CAD build for the part. Positions are in the model's coordinates, mm. A direction names the side the tool comes from. Give positions to 0.01 mm unless a question says otherwise; leave off trailing zeros. Loops run counter-clockwise (first coordinate to the right, second up) from the corner with the lowest first, then second, coordinate; pieces in that order, holes last.
```python
from build123d import *

# Parameters (mm, degrees)
ESQUISSE1_R        = 6.5
ESQUISSE1_R_2      = 6
ESQUISSE1_R_3      = 2.5
BOSS_EXTRU_1_DEPTH = 3
CONG_1_R           = 6


with BuildPart() as part:
    # Esquisse1 → Boss.-Extru.1 (new body)
    with BuildSketch(Plane.XY):
        with BuildLine():
            Line((0, 10), (20, 10))
            ThreePointArc((20, 10), (25.257311121, 8.506508084), (28.94427191, 4.472135955))
            Line((28.94427191, 4.472135955), (38.94427191, -15.527864045))
            ThreePointArc((38.94427191, -15.527864045), (34.472135955, -28.94427191), (21.05572809, -24.472135955))
            Line((21.05572809, -24.472135955), (13.819660113, -10))
            Line((13.819660113, -10), (6.180339887, -10))
            Line((6.180339887, -10), (-1.05572809, -24.472135955))
            ThreePointArc((-1.05572809, -24.472135955), (-14.472135955, -28.94427191), (-18.94427191, -15.527864045))
            Line((-18.94427191, -15.527864045), (-8.94427191, 4.472135955))
            ThreePointArc((-8.94427191, 4.472135955), (-5.257311121, 8.506508084), (0, 10))
        make_face()
        Circle(ESQUISSE1_R, mode=Mode.SUBTRACT)
        with Locations((20, 0)):
            Circle(ESQUISSE1_R_2, mode=Mode.SUBTRACT)
        with Locations((-10, -20)):
            Circle(ESQUISSE1_R_3, mode=Mode.SUBTRACT)
        with Locations((30, -20)):
            Circle(ESQUISSE1_R_3, mode=Mode.SUBTRACT)
    extrude(amount=BOSS_EXTRU_1_DEPTH)

    # Congé1
    cong_1_edges = [part.edges().sort_by_distance(p)[0] for p in [
        (6.180339887, -10, 1.5),
        (13.819660113, -10, 1.5),
    ]]
    fillet(cong_1_edges, radius=CONG_1_R)


solid = part.part
```
1. Saw through at B-B, the plane y = -26. List the corners of the cut face in (x, z).
Responses:
outline: (-18, 0) - (-2, 0) - (-2, 3) - (-18, 3) - close; (22, 0) - (38, 0) - (38, 3) - (22, 3) - close
2. Tool access for faces 5 (the face through (6.695, -10.921, 1.521)), 6 (the face through (-14.014, -5.668, 1.479)): list every direction of +Z, -Z, +X, -X, +Y, -Y with a clear straight run to the whole face (end or side of a thin tool).
Responses:
face 5: +Z, -Z, -Y
face 6: +Z, -Z, -X, +Y
3. Pull direction Y, two halves, no side cores. Call faces 1 (the face through (13.305, -10.921, 1.521)), 2 (the face through (-5.158, -3.955, 1.479)), 3 (the face through (10, 10, 1)), 4 (the face through (10.4, -9.7, 3)): released by +Y, released by -Y, zero draft, split by the parting line, or undercut.
Responses:
face 1: released by -Y
face 2: undercut
face 3: released by +Y
face 4: zero draft
4. Saw through at C-C, the plane y = 0. List the corners of the cut face in (x, z).
Responses:
outline: (-11.18, 0) - (-6.5, 0) - (-6.5, 3) - (-11.18, 3) - close; (6.5, 0) - (14, 0) - (14, 3) - (6.5, 3) - close; (26, 0) - (31.18, 0) - (31.18, 3) - (26, 3) - close
5. Drop a flat-ended pin along its axis: pin 1 (1.5 mm diameter, centred on x = -2.5, z = 2, fed in from +Y). Give the stop position or say it passes through.
Responses:
pin 1: stops at y = 9.85
6. Probe line 1 along X through (y, z) = (-19, 1.65); line 2 along X through (y, z) = (-22, 0.7); line 3 along X through (y, z) = (4, 2.55). List the from-to ranges inside material, lowest first.
Responses:
line 1: x = -19.95 to -12.29, -7.71 to 1.68, 18.32 to 27.71, 32.29 to 39.95
line 2: x = -19.8 to -11.5, -8.5 to 0.18, 19.82 to 28.5, 31.5 to 39.8
line 3: x = -9.18 to -5.12, 5.12 to 15.53, 24.47 to 29.18
7. Saw through at D-D, the plane x = -4.5. List the corners of the cut face in (y, z), and give its area (3 significant figures).
Responses:
outline: (-28.35, 0) - (-4.69, 0) - (-4.69, 3) - (-28.35, 3) - close; (4.69, 0) - (8.93, 0) - (8.93, 3) - (4.69, 3) - close
area: 83.7 mm2
